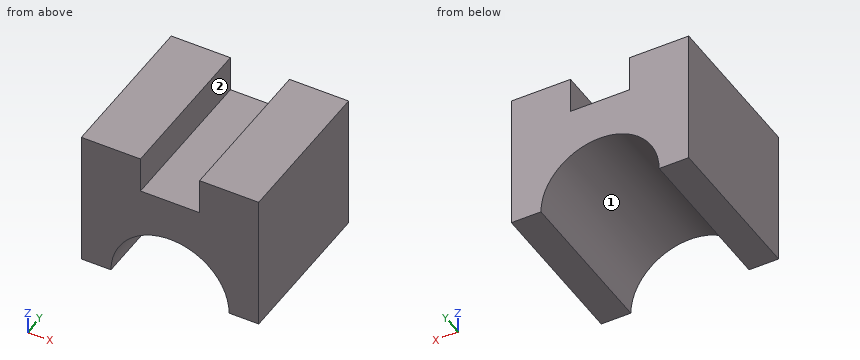
```python
from build123d import *

# Parameters (mm, degrees)
F1_DEPTH = 40


with BuildPart() as f1:
    # F0 (on Front) → F1 (new body)
    with BuildSketch(Plane.XZ):
        with BuildLine():
            Line((0, 35), (0, 0))
            Line((0, 0), (7.5, 0))
            ThreePointArc((7.5, 0), (22.5, 15), (37.5, 0))
            Line((37.5, 0), (45, 0))
            Line((45, 0), (45, 35))
            Line((45, 35), (30, 35))
            Line((30, 35), (30, 25.78854))
            Line((30, 25.78854), (15, 25.78854))
            Line((15, 25.78854), (15, 35))
            Line((15, 35), (0, 35))
        make_face()
    extrude(amount=F1_DEPTH)


solid = f1.part
```
Could you check a few things on this model? Use its own coordinates, in mm. Face numbers are marked on the shaded views. A direction names the side the tool comes from. Round coordinates to 2 decimals unless told otherwise and drop trailing zeros. Write each loop counter-clockwise with the first axis right and the second up, starting at its lowest first coordinate (ties: lowest second). Pieces come first, ordered by that corner, then holes. Notation, with made-up numbers: M 2.25,63 L 39.25,63 A25 cw 39.25,79 Z; hole C -19.75,-14.5 d8. An arc over 180 degrees is marked long. Answer in a Markdown table with one row per item. Add a question column.
Q1. Will this pin go through, and if not, where does the flat tip stop? pin 1 Ø8 at (y, z) = (-10, 18) entering from -X.
Q2. Imagine slicing it at D-D (x = 13.5). Please give me the cut outline in (y, z).
Q3. Imagine slicing it at C-C (x = 22.5). Please give me the cut outline in (y, z), then the cut area to 3 significant figures.
Q4. Imagine slicing it at A-A (z = 30.5). Please give me the cut outline in (x, y).
Q5. If I drill on line 1 (X direction, y = -26.5, z = 28); line 2 (X direction, y = -2.5, z = 12.5); line 3 (Z direction, x = 18, y = -5.5), over which ranges is the centre line in solid material (lowest first)? Write a range as from..to.
Q6. Imagine slicing it at B-B (y = -20). Please give me the cut outline in (x, z).
Q7. On a 3-axis mill with a long thin cutter (end or side, diameter ignored), from which of +Z, -Z, +X, -X, +Y, -Y can I reach the whole of each face in a straight line? I mean the marked faces 1 and 2. Say none if no direction works.
Values:
| question | item | result |
|---|---|---|
| 1 | pin 1 | x = 0 |
| 2 | outline | M -40,12 L 0,12 L 0,35 L -40,35 Z |
| 3 | outline | M -40,15 L 0,15 L 0,25.79 L -40,25.79 Z |
| 3 | area | 432 mm^2 |
| 4 | outline | M 0,-40 L 15,-40 L 15,0 L 0,0 Z; M 30,-40 L 45,-40 L 45,0 L 30,0 Z |
| 5 | line 1 | 0..15, 30..45 |
| 5 | line 2 | 0..14.21, 30.79..45 |
| 5 | line 3 | 14.31..25.79 |
| 6 | outline | M 0,0 L 7.5,0 A15 cw 37.5,0 L 45,0 L 45,35 L 30,35 L 30,25.79 L 15,25.79 L 15,35 L 0,35 Z |
| 7 | face 1 | -Z, +Y, -Y |
| 7 | face 2 | +Z, +Y, -Y |
